Work out the finished part from the listing and answer in its coordinate system (mm). A direction names the side the tool comes from. Round coordinates to 2 decimals unless told otherwise and drop trailing zeros. Order: outer loops, then holes, each group sorted by start corner. A loop starts at its lowest first (then second) coordinate and runs counter-clockwise, first axis right, second up. Notation, with made-up numbers: (80, 8.5) - (87, 8.5) arc R24 cw to (87, 32.5) - close; hole circle Ø6 at (76, 66). An arc over 180 degrees is marked (long way). Use CSV: the item, a comma, the result in double quotes.
from build123d import *

# Parameters (mm, degrees)
F1_R = 20
F3_T = -2


with BuildPart() as f2:
    # F2: sweep along a path in F0
    with BuildLine(Plane.XZ) as f2_path:
        Line((-160, 0), (-160, 50))
        ThreePointArc((-160, 50), (-136.5685424949, 106.5685424949), (-80, 130))
        Line((-80, 130), (60, 130))
    # F1 (on Top) → F2 (sweep)
    with BuildSketch(Plane.XY):
        with Locations((-160, 0)):
            Circle(F1_R)
    sweep(path=f2_path.line)

    # F3
    f3_openings = [f2.faces().sort_by_distance(p)[0] for p in [
        (-160, 0, 0),
        (60, 0, 130),
    ]]
    offset(amount=F3_T, openings=f3_openings)


solid = f2.part
(1) Find section B-B (x = -30.5). Determine the outline of the cut face in (y, z).
Findings below:
outline,"circle Ø40 at (0, 130); hole circle Ø36 at (0, 130)"
(2) Each of these flat-tipped pins is pushed along its axis until it touches: pin 1 (1 mm diameter, centred on x = -148.5, z = 125.5, fed in from +Y); pin 2 (6 mm diameter, centred on x = -113, y = -4, fed in from +Z); pin 3 (8 mm diameter, centred on x = 7, y = -15.5, fed in from +Z); pin 4 (6 mm diameter, centred on x = -108, y = -9, fed in from +Z). Where does it stop, or does it pass through?
Findings below:
pin 1,"passes through"
pin 2,"stops at z = 145.11"
pin 3,"stops at z = 146.36"
pin 4,"stops at z = 145.35"
(3) Find section D-D (y = -15). Determine the outline of the cut face in (x, z).
Findings below:
outline,"(-173.23, 0) - (-169.95, 0) - (-169.95, 50) arc R89.95 cw to (-80, 139.95) - (60, 139.95) - (60, 143.23) - (-80, 143.23) arc R93.23 ccw to (-173.23, 50) - close; (-150.05, 0) - (-146.77, 0) - (-146.77, 50) arc R66.77 cw to (-80, 116.77) - (60, 116.77) - (60, 120.05) - (-80, 120.05) arc R70.05 ccw to (-150.05, 50) - close"
(4) Find the intervals of material crossed by L1, parallel to Y at x = -160, z = 33.5; L2, parallel to Z at x = -99.5, y = 10; L3, parallel to Z at x = -99.5, y = -8, in increasing order. Write a range as from..to.
Findings below:
L1,"y = -20..-18, 18..20"
L2,"z = 109.57..112.04, 142.94..145.35"
L3,"z = 108.51..110.83, 144.13..146.38"
(5) Find section C-C (z = 42.5). Determine the outline of the cut face in (x, y).
Findings below:
outline,"circle Ø40 at (-160, 0); hole circle Ø36 at (-160, 0)"
(6) The mould has two halves that part along Y. Classify faces 3 (the cylindrical face through (-9.02, 0.88, 149.98)), 4 (the cylindrical face through (-9.02, 5.407, 112.831)), 5 (the flat face through (-178, 3, 0)), 6 (the cylindrical face through (-142.831, 5.407, 25.35)): released by +Y, released by -Y, zero draft, split by the parting line, or undercut.
Findings below:
face 3,"split by the parting line"
face 4,"undercut"
face 5,"zero draft"
face 6,"undercut"
(7) Find section A-A (y = 0). Determine the outline of the cut face in (x, z).
Findings below:
outline,"(-180, 0) - (-178, 0) - (-178, 50) arc R98 cw to (-80, 148) - (60, 148) - (60, 150) - (-80, 150) arc R100 ccw to (-180, 50) - close; (-142, 0) - (-140, 0) - (-140, 50) arc R60 cw to (-80, 110) - (60, 110) - (60, 112) - (-80, 112) arc R62 ccw to (-142, 50) - close"
(8) For faces 1 (the flat face through (60, -3, 112)), 2 (the cylindrical face through (-179.98, 0.88, 25.35)), determine the directions among +Z, -Z, +X, -X, +Y, -Y from which every point of the face is accessible in a straight line to the end or side of a thin tool.
Findings below:
face 1,"+Z, -Z, +X, +Y, -Y"
face 2,"-Z"
